Work out the finished part from the listing and answer in its coordinate system (mm). Face numbers are marked on the shaded views. A direction names the side the tool comes from. Round coordinates to 2 decimals unless told otherwise and drop trailing zeros. Write each loop counter-clockwise with the first axis right and the second up, starting at its lowest first coordinate (ties: lowest second). Pieces come first, ordered by that corner, then holes. Notation, with made-up numbers: (36.5, 3) -> (85.5, 3) arc R25 cw to (85.5, 37) -> close; hole circle Ø8 at (30, 57.5). An arc over 180 degrees is marked (long way). One line per question, with ' | ' between items. Start each with the question number.
```python
from build123d import *

# Parameters (mm, degrees)
SKETCH1_W           = 70
SKETCH1_H           = 20
BOSS_EXTRUDE1_DEPTH = 0.75
SKETCH2_W           = 7
SKETCH2_H           = 10
BOSS_EXTRUDE2_DEPTH = 6


with BuildPart() as part:
    # Sketch1 → Boss-Extrude1 (new, symmetric)
    with BuildSketch(Plane.XY):
        Rectangle(SKETCH1_W, SKETCH1_H)
    extrude(amount=BOSS_EXTRUDE1_DEPTH, both=True)

    # Sketch2 → Boss-Extrude2 (add)
    with BuildSketch(Plane.XY.offset(0.75)):
        with Locations((-31.5, 0)):
            Rectangle(SKETCH2_W, SKETCH2_H)
    extrude(amount=BOSS_EXTRUDE2_DEPTH)


solid = part.part
```
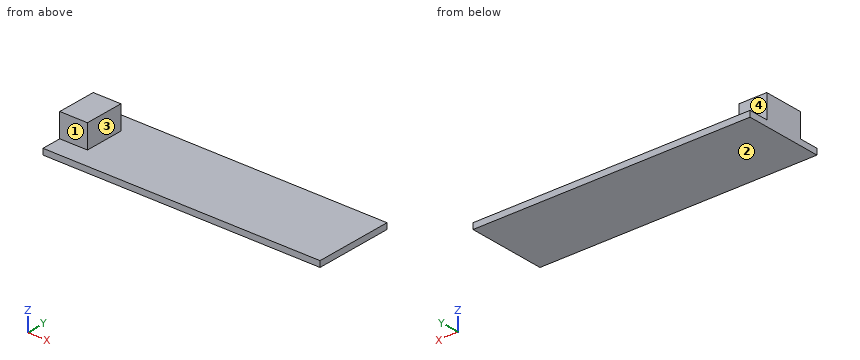
(1) A cutting plane is placed at A-A, the plane y = 1.5. Determine the outline of the cut face in (x, z).
(2) A cutting plane is placed at B-B, the plane x = -5. Determine the outline of the cut face in (y, z).
(3) A cutting plane is placed at C-C, the plane z = 3.25. Determine the outline of the cut face in (x, y).
(4) Given pin 1 Ø1.8 at (x, z) = (-31.5, 5) entering from +Y; pin 2 Ø5 at (x, y) = (-21.5, 4.5) entering from +Z; pin 3 Ø3 at (x, z) = (-32.5, 3) entering from -Y, each flat-ended and moving along its own axis, determine where each tip first touches the part or whether it passes through.
(5) Consider L1, parallel to X at y = -4.25, z = 3.75; L2, parallel to Z at x = 23, y = 6.5. Determine where each line is inside the solid, lowest interval first.
(6) For the marked faces 1, 2, 3 and 4, determine the directions among +Z, -Z, +X, -X, +Y, -Y from which every point of the face is accessible in a straight line to the end or side of a thin tool.
Returned:
1) outline: (-35, -0.75) -> (35, -0.75) -> (35, 0.75) -> (-28, 0.75) -> (-28, 6.75) -> (-35, 6.75) -> close
2) outline: (-10, -0.75) -> (10, -0.75) -> (10, 0.75) -> (-10, 0.75) -> close
3) outline: (-35, -5) -> (-28, -5) -> (-28, 5) -> (-35, 5) -> close
4) pin 1: y = 5 | pin 2: z = 0.75 | pin 3: y = -5
5) L1: -35 to -28 | L2: -0.75 to 0.75
6) face 1: +Z, +X, -X, -Y | face 2: -Z, +X, -X, +Y, -Y | face 3: +Z, +X, +Y, -Y | face 4: +Z, +X, -X, +Y
